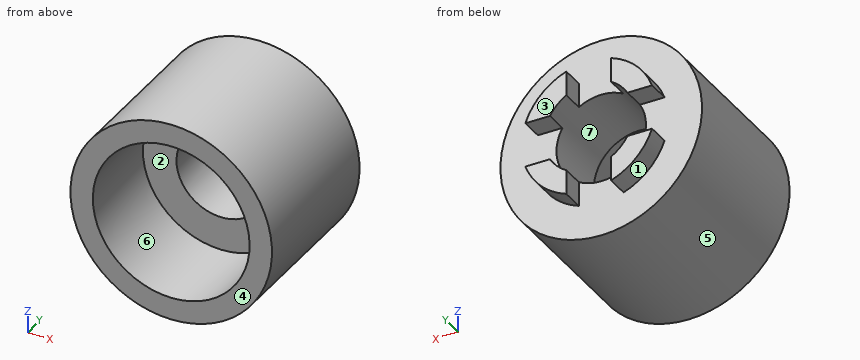
```python
from build123d import *

# Parameters (mm, degrees)
SKETCH2_R           = 28.575
SKETCH2_R_2         = 12.7
BOSS_EXTRUDE2_DEPTH = 50.8
SKETCH4_W           = 76.2
SKETCH4_H           = 12.7
CUT_EXTRUDE7_DEPTH  = 6.35
CIRPATTERN1_COUNT   = 2
CIRPATTERN1_ANGLE   = 90
SKETCH9_R           = 22.225
CUT_EXTRUDE8_DEPTH  = 25.4
CUT_EXTRUDE10_START = -6.35
SKETCH10_R          = 28.575
SKETCH10_R_2        = 19.05
CUT_EXTRUDE10_DEPTH = 6.35


with BuildPart() as part:
    # Sketch2 → Boss-Extrude2 (new body)
    with BuildSketch(Plane(origin=(0, 0, 0), x_dir=(1, 0, 0), z_dir=(0, 1, 0))):
        with Locations(Location((0, 0, 0), (0, 0, 270))):
            Circle(SKETCH2_R)
        with Locations(Location((0, 0, 0), (0, 0, 270))):
            Circle(SKETCH2_R_2, mode=Mode.SUBTRACT)
    extrude(amount=BOSS_EXTRUDE2_DEPTH)

    # Sketch4 → Cut-Extrude7 (cut)
    with BuildSketch(Plane(origin=(0, 50.8, 0), x_dir=(1, 0, 0), z_dir=(0, 1, 0))):
        Rectangle(SKETCH4_W, SKETCH4_H)
    cut_extrude7 = extrude(amount=-CUT_EXTRUDE7_DEPTH, mode=Mode.SUBTRACT)

    # CirPattern1: Cut-Extrude7 ×2 about axis
    cirpattern1_axis = Axis((0, 50.8, 0), (0, 1, 0))
    for i in range(1, CIRPATTERN1_COUNT):
        add(cut_extrude7.rotate(cirpattern1_axis, i * CIRPATTERN1_ANGLE / (CIRPATTERN1_COUNT - 1)), mode=Mode.SUBTRACT)

    # Sketch9 → Cut-Extrude8 (cut)
    with BuildSketch(Plane.XZ):
        with Locations(Location((0, 0, 0), (0, 0, 270))):
            Circle(SKETCH9_R)
    extrude(amount=-CUT_EXTRUDE8_DEPTH, mode=Mode.SUBTRACT)

    # Sketch10 → Cut-Extrude10 (cut)
    with BuildSketch(Plane(origin=(0, 50.8, 0), x_dir=(1, 0, 0), z_dir=(0, 1, 0)).offset(CUT_EXTRUDE10_START)):
        with Locations(Location((0, 0, 0), (0, 0, 90))):
            Circle(SKETCH10_R)
        Circle(SKETCH10_R_2, mode=Mode.SUBTRACT)
    extrude(amount=CUT_EXTRUDE10_DEPTH, mode=Mode.SUBTRACT)


solid = part.part
```
Model file for the job. Use its own axes, mm. Face numbers are marked on the shaded views. A direction names the side the tool comes from. Coordinates: 2 decimals unless noted, no trailing zeros. Order: outer loops, then holes, each group sorted by start corner. A loop starts at its lowest first (then second) coordinate and runs counter-clockwise, first axis right, second up. Notation, with made-up numbers: M 83,75.25 L 114,75.25 A33 cw 114,110.25 Z; hole C 42.5,78 d8. An arc over 180 degrees is marked long. Answer as CSV lines item,"result".
(1) 3-axis set-ups, long thin cutter, end or side, ignore diameter. For the marked faces 1, 2 and 3: which of +Z, -Z, +X, -X, +Y, -Y reach the whole face in a straight line?
Geometry says:
face 1,"-Z, -X, +Y"
face 2,"-Y"
face 3,"+Z, -Z, +X, -X, +Y"
(2) Band-saw the part on C-C, the plane y = 28. List the corners of the cut face in (x, z) (3 decimals), then the cut area to 3 significant figures.
Geometry says:
outline,"C 0,0 d57.15; hole C 0,0 d25.4"
area,"2,060 mm2"
(3) Flat gauge pins, fed straight in: pin 1 (3 mm diameter, centred on x = -15.5, z = 18.5, fed in from +Y); pin 2 (5 mm diameter, centred on y = 49, z = -15.5, fed in from -X); pin 3 (15 mm diameter, centred on x = 0, z = 0, fed in from +Y); pin 4 (6 mm diameter, centred on x = -9, y = 29.5, fed in from -Z). Where does each tip first touch, or does it go through?
Geometry says:
pin 1,"stops at y = 44.45"
pin 2,"stops at x = -13.92"
pin 3,"passes through"
pin 4,"stops at z = -27.94"
(4) Band-saw the part on B-B, the plane x = 0. List the corners of the cut face in (y, z) (3 decimals).
Geometry says:
outline,"M 0,-28.575 L 44.45,-28.575 L 44.45,-12.7 L 25.4,-12.7 L 25.4,-22.225 L 0,-22.225 Z; M 0,22.225 L 25.4,22.225 L 25.4,12.7 L 44.45,12.7 L 44.45,28.575 L 0,28.575 Z"
(5) Pull direction Z, two halves, no side cores. Call the marked faces 4, 5, 6 and 7: +Z half, -Z half, draft (parallel to the pull), parting line (faces both ways), or undercut.
Geometry says:
face 4,"draft"
face 5,"parting line"
face 6,"undercut"
face 7,"undercut"
(6) Wall check: line 1 along X through (y, z) = (31.75, 0) (3 decimals); line 2 along X through (y, z) = (8.25, 0) (3 decimals); line 3 along Y through (x, z) = (-18, -15). Give the ranges that are in metal, low to high.
Geometry says:
line 1,"x = -28.575 to -12.7, 12.7 to 28.575"
line 2,"x = -28.575 to -22.225, 22.225 to 28.575"
line 3,"y = 0 to 44.45"
(7) Band-saw the part on D-D, the plane x = -15. List the corners of the cut face in (y, z).
Geometry says:
outline,"M 0,-24.32 L 44.45,-24.32 L 44.45,-11.74 L 50.8,-11.74 L 50.8,-6.35 L 44.45,-6.35 L 44.45,6.35 L 50.8,6.35 L 50.8,11.74 L 44.45,11.74 L 44.45,24.32 L 0,24.32 L 0,16.4 L 25.4,16.4 L 25.4,-16.4 L 0,-16.4 Z"
(8) Band-saw the part on A-A, the plane z = 0. List the corners of the cut face in (x, y) (3 decimals).
Geometry says:
outline,"M -28.575,0 L -22.225,0 L -22.225,25.4 L -12.7,25.4 L -12.7,44.45 L -28.575,44.45 Z; M 12.7,25.4 L 22.225,25.4 L 22.225,0 L 28.575,0 L 28.575,44.45 L 12.7,44.45 Z"
